Verification items for the finished model (mm, model axes). Face numbers are marked on the shaded views. A direction names the side the tool comes from. Coordinates: 2 decimals unless noted, no trailing zeros. Loops run counter-clockwise (first coordinate to the right, second up) from the corner with the lowest first, then second, coordinate; pieces in that order, holes last. Notation, with made-up numbers: (26.25, -31) -> (61.25, -31) arc R27 ccw to (61.25, 0) -> close; hole circle Ø7 at (66.5, 20.5). An arc over 180 degrees is marked (long way). Write item = value, one per line.
```python
from build123d import *

# Parameters (mm, degrees)
SKETCH_1_R               = 22.5
SKETCH_1_R_2             = 2
EXTRUDE_1_DEPTH          = 5
SKETCH_2_R               = 10.25
CUT_EXTRUDE_1_DEPTH      = 1
CUT_EXTRUDE_2_DEPTH      = 33.210246817
CUT_EXTRUDE_2_DEPTH_BACK = 33.210246817
SKETCH_3_W               = 12
SKETCH_3_H               = 3
SKETCH_4_R               = 1
CUT_EXTRUDE_3_DEPTH      = 33.210246817


with BuildPart() as part:
    # 草图1 → 凸台-拉伸1 (new body)
    with BuildSketch(Plane(origin=(0, 0, 0), x_dir=(1, 0, 0), z_dir=(0, 1, 0))):
        with Locations(Location((0, 0, 0), (0, 0, 270))):
            Circle(SKETCH_1_R)
        with Locations(Location((18.5, 0, 0), (0, 0, 270))):
            Circle(SKETCH_1_R_2, mode=Mode.SUBTRACT)
        with Locations(Location((-18.5, 0, 0), (0, 0, 90))):
            Circle(SKETCH_1_R_2, mode=Mode.SUBTRACT)
    extrude(amount=EXTRUDE_1_DEPTH)

    # 草图2 → 切除-拉伸1 (cut)
    with BuildSketch(Plane(origin=(0, 0, 0), x_dir=(1, 0, 0), z_dir=(0, 1, 0))):
        with Locations(Location((0, 0, 0), (0, 0, 270))):
            Circle(SKETCH_2_R)
    extrude(amount=CUT_EXTRUDE_1_DEPTH, mode=Mode.SUBTRACT)

    # 草图3 → 切除-拉伸2 (cut, two sides: drawn at the far end of the back side and taken through both)
    with BuildSketch(Plane.XY.offset(-CUT_EXTRUDE_2_DEPTH_BACK)):
        with Locations((0, 1.5)):
            Rectangle(SKETCH_3_W, SKETCH_3_H)
    extrude(amount=CUT_EXTRUDE_2_DEPTH + CUT_EXTRUDE_2_DEPTH_BACK, mode=Mode.SUBTRACT)

    # 草图4 → 切除-拉伸3 (cut, through all)
    with BuildSketch(Plane(origin=(0, 5, 0), x_dir=(1, 0, 0), z_dir=(0, 1, 0))):
        with Locations(Location((13.081475452, 13.081475452, 0), (0, 0, 270))):
            Circle(SKETCH_4_R)
        with Locations(Location((13.081475452, -13.081475452, 0), (0, 0, 270))):
            Circle(SKETCH_4_R)
        with Locations(Location((-13.081475452, 13.081475452, 0), (0, 0, 270))):
            Circle(SKETCH_4_R)
        with Locations(Location((-13.081475452, -13.081475452, 0), (0, 0, 270))):
            Circle(SKETCH_4_R)
    extrude(amount=-CUT_EXTRUDE_3_DEPTH, mode=Mode.SUBTRACT)


solid = part.part
```
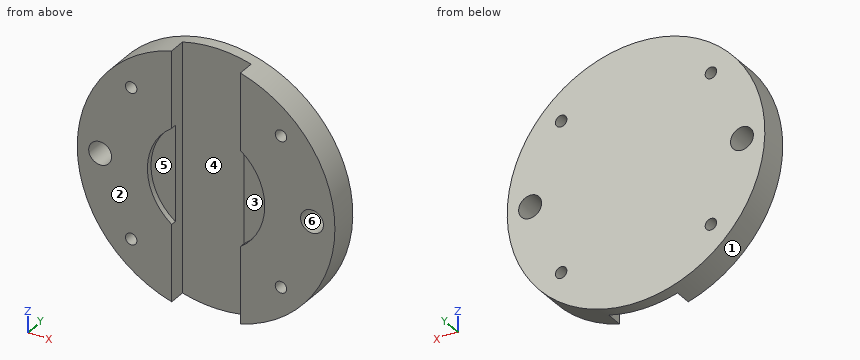
1) Tool access check on the marked faces 4, 5 and 6. Record the directions out of +Z, -Z, +X, -X, +Y, -Y that give a thin tool (end or side, any length) a straight path to the whole face; none if there is none.
Ans:
face_4 = +Z, -Z, -Y
face_5 = -Y
face_6 = +Y, -Y
2) Release check for a two-part mould opening along X. For the marked faces 1, 2 and 3 record: pulls with the +X half, pulls with the -X half, needs draft (parallel to the pull), parting line crosses it, or undercut.
Ans:
face_1 = parting line crosses it
face_2 = needs draft
face_3 = undercut
3) Depth check by flat-ended pin: pin 1 Ø6 at (x, z) = (0, 10.5) entering from -Y; pin 2 Ø3 at (x, z) = (18.5, 0) entering from -Y; pin 3 Ø3 at (y, z) = (3.5, 10.5) entering from -X; pin 4 Ø2 at (x, z) = (7, -0.5) entering from -Y. Enter the tip coordinate at first touch or a pass-through.
Ans:
pin_1 = 3
pin_2 = through
pin_3 = -20.62
pin_4 = 1
4) Material ranges on line 1 (X direction, y = 4.55, z = -13); line 2 (X direction, y = 4.75, z = -1); line 3 (X direction, y = 2.35, z = -1), recorded low to high.
Ans:
line_1 = -18.36 to -14.08, -12.08 to 12.08, 14.08 to 18.36
line_2 = -22.48 to -20.23, -16.77 to 16.77, 20.23 to 22.48
line_3 = -22.48 to -20.23, -16.77 to -6, 6 to 16.77, 20.23 to 22.48
5) Sectioned sample at D-D, the plane z = 15.5. Record the cut outline in (x, y).
Ans:
outline = (-16.31, 0) -> (-6, 0) -> (-6, 3) -> (6, 3) -> (6, 0) -> (16.31, 0) -> (16.31, 5) -> (-16.31, 5) -> close
6) Sectioned sample at C-C, the plane y = 4.2. Record the cut outline in (x, z).
Ans:
outline = circle Ø45 at (0, 0); hole circle Ø4 at (-18.5, 0); hole circle Ø2 at (-13.08, -13.08); hole circle Ø2 at (-13.08, 13.08); hole circle Ø2 at (13.08, -13.08); hole circle Ø2 at (13.08, 13.08); hole circle Ø4 at (18.5, 0)
7) Sectioned sample at A-A, the plane z = 0. Record the cut outline in (x, y).
Ans:
outline = (-22.5, 0) -> (-20.5, 0) -> (-20.5, 5) -> (-22.5, 5) -> close; (-16.5, 0) -> (-10.25, 0) -> (-10.25, 1) -> (-6, 1) -> (-6, 3) -> (6, 3) -> (6, 1) -> (10.25, 1) -> (10.25, 0) -> (16.5, 0) -> (16.5, 5) -> (-16.5, 5) -> close; (20.5, 0) -> (22.5, 0) -> (22.5, 5) -> (20.5, 5) -> close
8) Sectioned sample at B-B, the plane x = -18.5. Record the cut outline in (y, z).
Ans:
outline = (0, -12.81) -> (5, -12.81) -> (5, -2) -> (0, -2) -> close; (0, 2) -> (5, 2) -> (5, 12.81) -> (0, 12.81) -> close
